Here's the drawing with two shaded views (mm, measured from the low corner). I have some questions. Give positions to 0.01 mm unless a question says otherwise; leave off trailing zeros. Order: outer loops, then holes, each group sorted by start corner. A loop starts at its lowest first (then second) coordinate and runs counter-clockwise, first axis right, second up. Notation, with made-up numbers: (-30.75, -12) - (-8.75, -12) arc R27 cw to (-8.75, 14) - close; hole circle Ø8 at (-8.5, -2). An arc over 180 degrees is marked (long way). Use one line per item in the form item = value. Start each with the question number.
1) For pin 1 (3 mm diameter, centred on y = 4.5, z = 8, fed in from +X); pin 2 (1.8 mm diameter, centred on x = 26, z = 5, fed in from +Y), each with a flat end and sliding along its axis, tell me the tip position at first contact or that it passes through.
2) Please list where these lines run through material, in increasing order: probe 1 along Z at (x, y) = (4, 1.2); probe 2 along X at (y, z) = (2.2, 5); probe 3 along Y at (x, z) = (15, 4).
3) We'd pull the mould along Z, two halves only. Please class the marked faces 1, 2, 3 and 4: released by +Z, released by -Z, zero draft, split by the parting line, or undercut.
4) Suppose I cut it at A-A, the plane x = 4. Write out the boundary of the cut face in (y, z), and give its area (4 significant figures).
5) Suppose I cut it at B-B, the plane y = 3.55. Write out the boundary of the cut face in (x, z).
6) Suppose I cut it at D-D, the plane z = 8.5. Write out the boundary of the cut face in (x, y) (3 decimals).
7) Suppose I cut it at C-C, the plane y = 0.3. Write out the boundary of the cut face in (x, z).
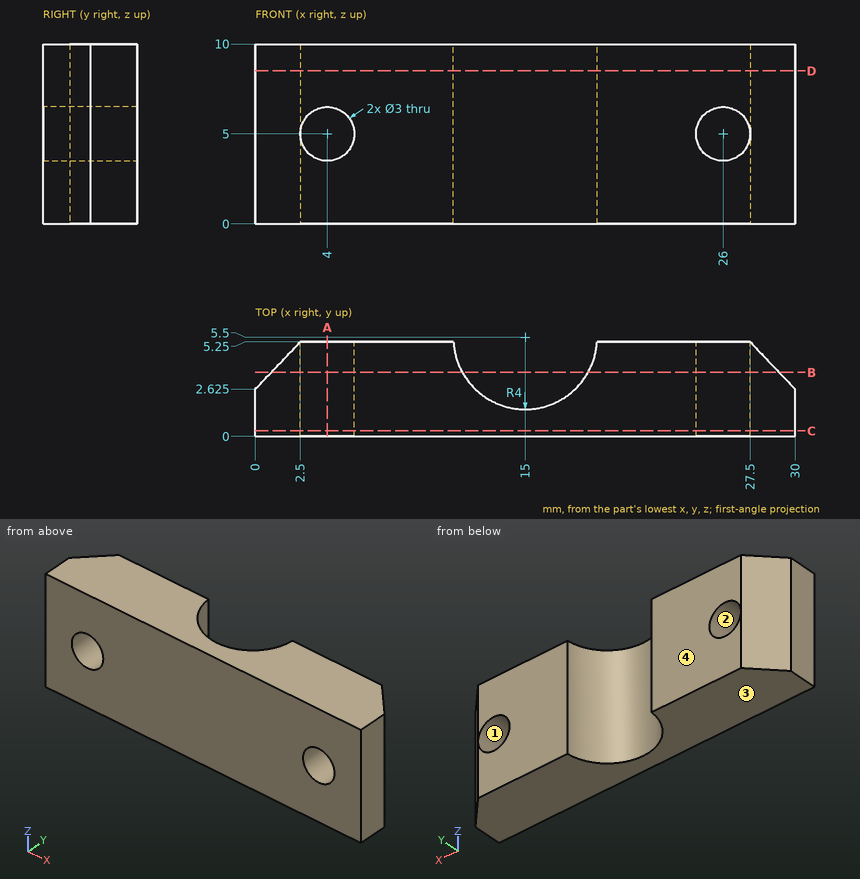
Result sheet:
q1.pin_1 = 29.64
q1.pin_2 = through
q2.probe_1 = 0 to 3.5, 6.5 to 10
q2.probe_2 = 0 to 2.5, 5.5 to 12.74, 17.26 to 24.5, 27.5 to 30
q2.probe_3 = 0 to 1.5
q3.face_1 = undercut
q3.face_2 = undercut
q3.face_3 = released by -Z
q3.face_4 = zero draft
q4.outline = (0, 0) - (5.25, 0) - (5.25, 3.5) - (0, 3.5) - close; (0, 6.5) - (5.25, 6.5) - (5.25, 10) - (0, 10) - close
q4.area = 36.75 mm²
q5.outline = (0.88, 0) - (11.51, 0) - (11.51, 10) - (0.88, 10) - close; (18.49, 0) - (29.12, 0) - (29.12, 10) - (18.49, 10) - close; hole circle Ø3 at (4, 5); hole circle Ø3 at (26, 5)
q6.outline = (0, 0) - (30, 0) - (30, 2.625) - (27.5, 5.25) - (18.992, 5.25) arc R4 cw to (11.008, 5.25) - (2.5, 5.25) - (0, 2.625) - close
q7.outline = (0, 0) - (30, 0) - (30, 10) - (0, 10) - close; hole circle Ø3 at (4, 5); hole circle Ø3 at (26, 5)
